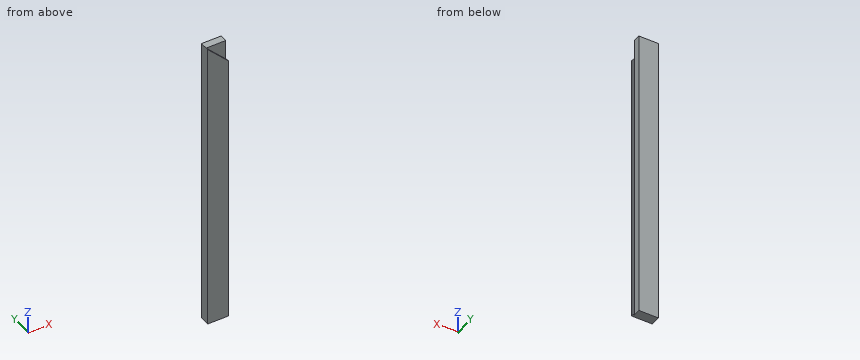
```python
from build123d import *

# Parameters (mm, degrees)
F1_DEPTH = 762
F3_DEPTH = 6.35


with BuildPart() as f1:
    # F0 (on Top) → F1 (new body)
    with BuildSketch(Plane.XY):
        Polygon((23.8125, -6.35), (23.8125, 12.7), (-26.9875, 12.7), (-26.9875, -12.7), (26.9875, -12.7), (26.9875, -6.35), align=None)
    extrude(amount=F1_DEPTH)

    # F2 (on face) → F3 (cut)
    with BuildSketch(Plane.XZ.offset(12.7)):
        Polygon((26.9875, 762), (-26.9875, 762), (26.9875, 708.025), align=None)
    extrude(amount=-F3_DEPTH, mode=Mode.SUBTRACT)


solid = f1.part
```
Read the model definition and answer for the solid it produces. Units are mm, in the model's axes. Round coordinates to 2 decimals unless told otherwise and drop trailing zeros. Write each loop counter-clockwise with the first axis right and the second up, starting at its lowest first coordinate (ties: lowest second). Pieces come first, ordered by that corner, then holes. Notation, with made-up numbers: (0.5, 2) - (28.5, 2) arc R20 cw to (28.5, 34) - close; hole circle Ø10 at (-37, 85). An arc over 180 degrees is marked (long way). One line per item, written item: value.
Q1. Each of these flat-tipped pins is pushed along its axis until it touches: P1, Ø2.5, axis at x = 25.5, z = 398, coming from the +Y side; P2, Ø6, axis at y = 3.5, z = 499.5, coming from the +X side. Where does it stop, or does it pass through?
The answers:
P1: stops at y = -6.35
P2: stops at x = 23.81
Q2. Find section B-B (y = -1.75). Determine the outline of the cut face in (x, z), and give its area (3 significant figures).
The answers:
outline: (-26.99, 0) - (23.81, 0) - (23.81, 762) - (-26.99, 762) - close
area: 38,700 mm2
Q3. Straight lines are drawn through the part: line 1 (X direction, y = 1, z = 130.5); line 2 (Y direction, x = 10, z = 727); line 3 (Z direction, x = -11.5, y = -7.5). For each, find the intervals that lie inside material, in ascending order. Write a range as from..to.
The answers:
line 1: x = -26.99..23.81
line 2: y = -6.35..12.7
line 3: z = 0..746.51
Q4. Find section A-A (z = 265). Determine the outline of the cut face in (x, y), and give its area (3 significant figures).
The answers:
outline: (-26.99, -12.7) - (26.99, -12.7) - (26.99, -6.35) - (23.81, -6.35) - (23.81, 12.7) - (-26.99, 12.7) - close
area: 1,310 mm2
